Check sheet for the modelled part. Datum: model origin and axes. Units: mm. Give positions to 0.01 mm unless a question says otherwise; leave off trailing zeros. Write each loop counter-clockwise with the first axis right and the second up, starting at its lowest first coordinate (ties: lowest second). Pieces come first, ordered by that corner, then holes.
from build123d import *

# Parameters (mm, degrees)
SKETCH1_W           = 15
SKETCH1_H           = 496.82
BOSS_EXTRUDE1_DEPTH = 4
SKETCH2_R           = 3
CUT_EXTRUDE1_DEPTH  = 8
CHAMFER1_SIZE       = 20
CHAMFER1_SIZE2      = 7.677280701
LPATTERN1_COUNT     = 6
LPATTERN1_PITCH     = 80
CHAMFER3_SIZE       = 3


with BuildPart() as part:
    # Sketch1 → Boss-Extrude1 (new, symmetric)
    with BuildSketch(Plane.XY):
        Rectangle(SKETCH1_W, SKETCH1_H)
    extrude(amount=BOSS_EXTRUDE1_DEPTH, both=True)

    # Sketch2 → Cut-Extrude1 (cut)
    with BuildSketch(Plane.XY.offset(4)):
        with Locations((0, 178.95225561)):
            Circle(SKETCH2_R)
    cut_extrude1 = extrude(amount=-CUT_EXTRUDE1_DEPTH, mode=Mode.SUBTRACT)

    # Chamfer1
    chamfer1_edges = [part.edges().sort_by_distance(p)[0] for p in [
        (0, -248.41, -4),
    ]]
    chamfer1_side = [part.faces().sort_by_distance(p)[0] for p in [
        (0, -0.68153803, -4),
    ]]
    chamfer(chamfer1_edges, length=CHAMFER1_SIZE, length2=CHAMFER1_SIZE2, reference=chamfer1_side[0])

    # LPattern1: Cut-Extrude1 ×6
    with Locations(*[(0, -i * LPATTERN1_PITCH, 0) for i in range(1, LPATTERN1_COUNT)]):
        add(cut_extrude1, mode=Mode.SUBTRACT)

    # Chamfer3
    chamfer3_edges = [part.edges().sort_by_distance(p)[0] for p in [
        (-3, 178.95225561, -4),
        (-3, 98.95225561, -4),
        (-3, 18.95225561, -4),
        (-3, -61.04774439, -4),
        (-3, -141.04774439, -4),
        (-3, -221.04774439, -4),
    ]]
    chamfer(chamfer3_edges, length=CHAMFER3_SIZE)


solid = part.part
1) Scan lines: L1, parallel to X at y = -139.5, z = -0.75; L2, parallel to Z at x = 1.5, y = -225.5. Record each from-to range of solid material in increasing order.
2) Sectioned sample at A-A on z = 2. Record the boundary of the cut face in (x, y), then the cut area to 3 significant figures.
3) Gauge pin test, flat ends, axial feed: pin 1 (8 mm diameter, centred on x = 0, y = -61.05, fed in from +Z); pin 2 (7 mm diameter, centred on x = 0, y = -141.05, fed in from -Z). Record the tip position at first contact, or that the pin passes through.
4) Draft check along X on faces 1 (the conical face through (-0.41, -137.929, -1.146)), 2 (the flat face through (7.5, -3, 0)), 3 (the conical face through (1.452, 96.162, -1.146)), 4 (the flat face through (0, 248.41, 0)). Enter one of: +X half, -X half, draft (parallel to the pull), parting line (faces both ways), or undercut.
5) Sectioned sample at B-B on x = 0. Give the number of separate pieces and of enclosed holes in the cut face, then the cut area to 3 significant figures.
Answers below:
1. L1: x = -7.5 to -2.57, 2.57 to 7.5
1. L2: z = -2.7 to 4
2. outline: (-7.5, -244.04) - (7.5, -244.04) - (7.5, 248.41) - (-7.5, 248.41) - close; hole circle Ø6 at (0, -221.05); hole circle Ø6 at (0, -141.05); hole circle Ø6 at (0, -61.05); hole circle Ø6 at (0, 18.95); hole circle Ø6 at (0, 98.95); hole circle Ø6 at (0, 178.95)
2. area: 7,220 mm2
3. pin 1: stops at z = 4
3. pin 2: stops at z = -1.5
4. face 1: undercut
4. face 2: +X half
4. face 3: undercut
4. face 4: draft
5. separate pieces: 7
5. enclosed holes: 0
5. area: 3,560 mm2
